Can you work these out from the drawing? Everything is in mm from the part's minimum corner. Coordinates: 2 decimals unless noted, no trailing zeros. Loops run counter-clockwise (first coordinate to the right, second up) from the corner with the lowest first, then second, coordinate; pieces in that order, holes last. Notation, with made-up numbers: (13, 19.25) - (24, 19.25) arc R24 ccw to (24, 33.25) - close; hole circle Ø4 at (73.25, 1.5). An arc over 180 degrees is marked (long way). One line per question, with ' | ' between items. Start each with the question number.
1. Please list where this line runs through material, in increasing order: L1, parallel to X at y = 2.05, z = 11. Write a range as [from, to].
2. I want a section at A-A, the plane z = 289. Write out the boundary of the cut face in (x, y).
3. I want a section at B-B, the plane x = 262. Count the separate pieces of the cut face and the enclosed holes in it, then the cut area to 3 significant figures.
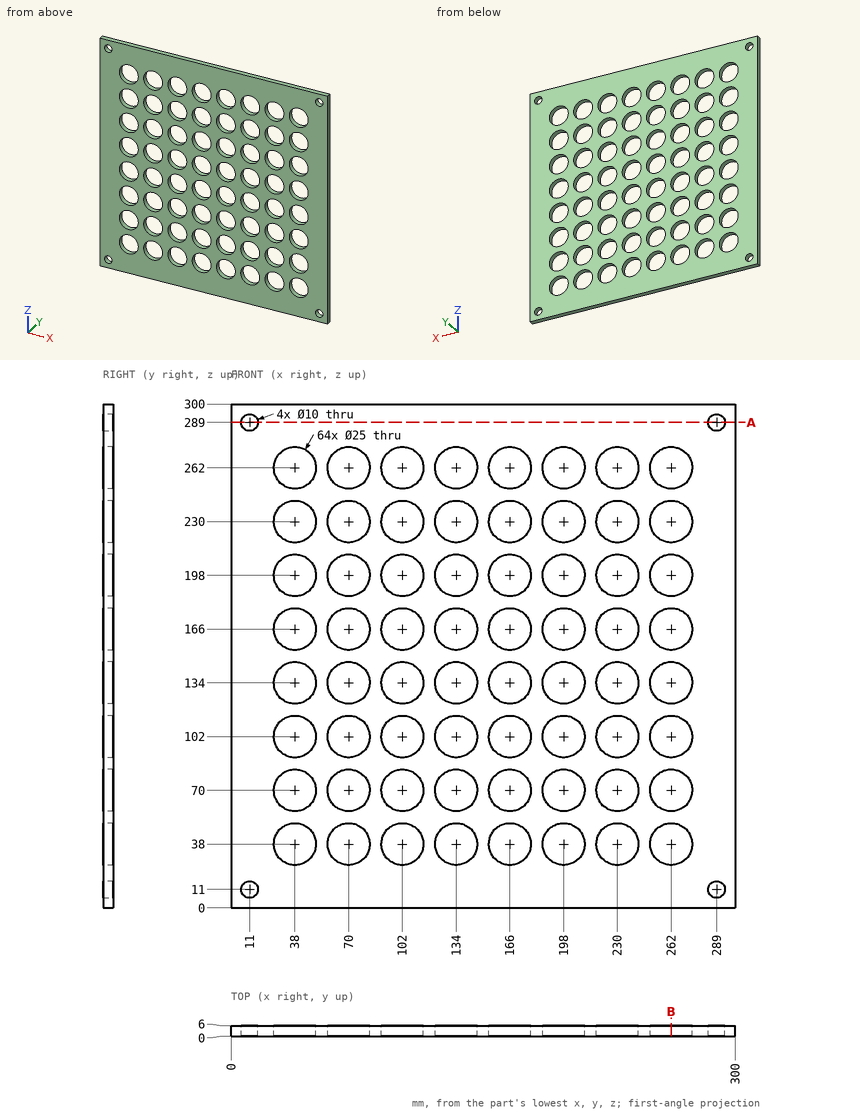
Results are:
1) L1: x = [0, 6], [16, 284], [294, 300]
2) outline: (0, 0) - (6, 0) - (6, 6) - (0, 6) - close; (16, 0) - (284, 0) - (284, 6) - (16, 6) - close; (294, 0) - (300, 0) - (300, 6) - (294, 6) - close
3) separate pieces: 9 | enclosed holes: 0 | area: 600 mm2
